Input: part model. Units: mm. Frame: model coordinates. A direction names the side the tool comes from. Coordinates: 2 decimals unless noted, no trailing zeros. Order: outer loops, then holes, each group sorted by start corner. A loop starts at its lowest first (then second) coordinate and runs counter-clockwise, first axis right, second up. Notation, with made-up numbers: (87.25, -34) -> (133.25, -34) arc R26 cw to (133.25, -15) -> close; hole circle Ø5 at (-31.5, 72). An arc over 180 degrees is marked (long way). Write each question's results on one line, items separated by ' | '.
Autodesk Inventor part; units mm, degrees
ref_plane "YZ Plane" through (0, 0, 0) normal (1, 0, 0) x (0, 1, 0)
ref_plane "XZ Plane" through (0, 0, 0) normal (0, 1, 0) x (-1, 0, 0)
ref_plane "XY Plane" through (0, 0, 0) normal (0, 0, 1) x (1, 0, 0)
sketch "Sketch1" plane through (0, 0, 0) normal (0, 1, 0) x (-1, 0, 0)
  line L0 (0, 0) -> (1.1, 0)
  line L1 (1.1, 0) -> (1.1, -2)
  line L2 (1.1, -2) -> (9.6, -2)
  line L3 (9.6, -2) -> (9.6, 0)
  line L4 (9.6, 0) -> (10.7, 0)
  line L5 (10.7, 0) -> (10.7, -29)
  line L6 (10.7, -29) -> (9.6, -29)
  line L7 (9.6, -29) -> (9.6, -27)
  line L8 (9.6, -27) -> (1.1, -27)
  line L9 (1.1, -27) -> (1.1, -29)
  line L10 (1.1, -29) -> (0, -29)
  line L11 (0, -29) -> (0, 0)
  dimension "d7" = 8.5
  dimension "d8" = 8.5
  dimension "d9" = 2
  dimension "d10" = 2
  dimension "d11" = 10.7
  dimension "d12" = 1.1
  dimension "d13" = 1.1
  dimension "d14" = 29
extrude "Extrusion1" add sketch "Sketch1" along normal blind 4.25
sketch "Sketch4" plane through (-9.6, 0, -2) normal (0, 0, 1) x (1, 0, 0)
  line L0 (8.5, 4.25) -> (0, 4.25)
  line L1 (8.5, 4.25) -> (9.6, 4.25)
  arc A0 (8.5, 4.25) -> (0, 4.25) centre (4.25, 4.25) ccw
  point P0 (9.6, 0)
extrude "Extrusion2" add sketch "Sketch4" along normal blind 10
sketch "Sketch5" plane through (-9.6, 0, -2) normal (0, 0, 1) x (1, 0, 0)
  line L0 (0, 0) -> (8.5, 0)
  line L1 (9.6, 4.25) -> (8.5, 4.25)
  line L2 (0, 0) -> (8.5, 0)
  line L3 (8.5, 0) -> (8.5, 4.25)
  line L4 (8.5, 4.25) -> (0, 4.25)
  line L5 (0, 4.25) -> (0, 0)
  point P0 (9.6, 0)
extrude "Extrusion3" add sketch "Sketch5" along normal blind 10
sketch "Sketch6" plane through (-9.6, 0, 8) normal (0, 0, 1) x (1, 0, 0)
  arc A0 (8.5, 4.25) -> (0, 4.25) centre (4.25, 4.25) ccw
  circle A1 centre (4.25, 4.25) radius 1.25
  point P0 (9.6, 0)
  dimension "d24" = 2.5
extrude "Extrusion4" cut sketch "Sketch6" against normal blind 10
sketch "Sketch9" plane through (-1.1, 0, -27) normal (0, 0, -1) x (-1, 0, 0)
  line L0 (0, 4.25) -> (8.5, 4.25)
  arc A0 (8.5, 4.25) -> (0, 4.25) centre (4.25, 4.25) ccw
  point P0 (-1.1, 0)
extrude "Extrusion6" add sketch "Sketch9" along normal blind 10
sketch "Sketch10" plane through (-1.1, 0, -27) normal (0, 0, -1) x (-1, 0, 0)
  line L0 (8.5, 4.25) -> (9.6, 4.25)
  line L1 (0, 0) -> (8.5, 0)
  line L2 (8.5, 0) -> (8.5, 4.25)
  line L3 (8.5, 4.25) -> (0, 4.25)
  line L4 (0, 4.25) -> (0, 0)
  point P0 (-1.1, 0)
extrude "Extrusion7" add sketch "Sketch10" along normal blind 10
sketch "Sketch11" plane through (-1.1, 0, -37) normal (0, 0, -1) x (-1, 0, 0)
  arc A0 (5.5, 4.25) -> (3, 4.25) centre (4.25, 4.25) ccw
  line L0 (8.5, 4.25) -> (5.5, 4.25)
  circle A1 centre (4.25, 4.25) radius 1.25
  point P0 (-1.1, 0)
extrude "Extrusion8" cut sketch "Sketch11" against normal blind 10
chamfer "Chamfer1" distance 2 angle 45 1 edges at (-5.35, 8.5, -2)
chamfer "Chamfer2" distance 2 angle 45 1 edges at (-5.35, 8.5, -27)
fillet "Fillet1" radius 1.1 4 edges at (0, 2.125, 0) (0, 2.125, -29) (-10.7, 2.125, 0) (-10.7, 2.125, -29)
properties part number "tracks_center_ver2"
(1) Reachability of faces 1 (the face through (-1.1, 2, -33)), 2 (the face through (-5.3, 6.8, -1.7)), 3 (the face through (-1.1, 2, 4)) from +Z, -Z, +X, -X, +Y, -Y: full face, straight path, thin tool, end or side. Return the list, or none.
Return value:
face 1: -Z, +X, +Y, -Y | face 2: +Y | face 3: +Z, +X, +Y, -Y
(2) Mould query, pull axis Y, two halves, no side actions, for faces 4 (the face through (-5.08, 3.03, -32.07)), 5 (the face through (-5.4, 8.5, 3.9)), 6 (the face through (-4, 3, 8)). Classes: +Y half, -Y half, draft (parallel to the pull), parting line (faces both ways), or undercut.
Return value:
face 4: undercut | face 5: +Y half | face 6: draft
(3) Line query: line 1 along Y through (x, z) = (-5.35, 4.5); line 2 along X through (y, z) = (4.25, -33.25); line 3 along Z through (x, y) = (-6.5, 5.25). Output: solid intervals per line, ascending. Write a range as from..to.
Return value:
line 1: 0..3, 5.5..8.5 | line 2: -9.6..-6.6, -4.1..-1.1 | line 3: -37..-27, -2..8
(4) Cut plane D-D, the plane z = -17.5. Return loops of the section in (x, y), plus the area to 3 significant figures.
Return value:
outline: (-10.7, 0) -> (0, 0) -> (0, 4.25) -> (-10.7, 4.25) -> close | area: 45.5 mm2
(5) Cut plane B-B, the plane z = 4. Return loops of the section in (x, y).
Return value:
outline: (-9.6, 0) -> (-1.1, 0) -> (-1.1, 4.25) arc R4.25 ccw to (-9.6, 4.25) -> close; hole circle Ø2.5 at (-5.35, 4.25)
(6) Cut plane A-A, the plane x = -5.35. Return loops of the section in (y, z), plus the area to 3 significant figures.
Return value:
outline: (0, -37) -> (3, -37) -> (3, -27) -> (4.25, -27) -> (4.25, -2) -> (3, -2) -> (3, 8) -> (0, 8) -> close; (5.5, -37) -> (8.5, -37) -> (8.5, -29) -> (6.5, -27) -> (5.5, -27) -> close; (5.5, -2) -> (6.5, -2) -> (8.5, 0) -> (8.5, 8) -> (5.5, 8) -> close | area: 222 mm2
(7) Pin query (flat end, axial travel): P1, Ø1.3, axis at y = 1, z = -33.5, coming from the -X side; P2, Ø1, axis at x = -2, z = -2.5, coming from the +Y side; P3, Ø1.5, axis at x = -5.35, y = 4.25, coming from the -Z side. Return the tip coordinate at first contact, or that it passes through.
Return value:
P1: x = -9.6 | P2: y = 4.25 | P3: z = -27
